For this review, take the finished solid that the model builds, in its own axes (mm). A direction names the side the tool comes from. Coordinates: 2 decimals unless noted, no trailing zeros. Loops run counter-clockwise (first coordinate to the right, second up) from the corner with the lowest first, then second, coordinate; pieces in that order, holes last.
1. Take a section at B-B, the plane x = -6.5. State the section outline as (y, z) points.
2. Clearance check with flat-ended pins moving along their axes: P1, Ø7.5, axis at y = 14, z = 48, coming from the +X side; P2, Ø1, axis at x = -1.5, z = 45, coming from the +Y side; P3, Ø10, axis at x = 8, y = -21, coming from the -Z side. State where each tip first meets the part, or that it passes through.
3. Machinability: for faces 1 (the face through (22.87, 19.61, 81.98)), 2 (the face through (15, 2.635, 16)), 3 (the face through (15, -20, 70)), 4 (the face through (14.45, -30.89, 41.74)), which of the approach directions +Z, -Z, +X, -X, +Y, -Y give a long, thin tool a straight path to every point of the face, cutting with its end or side? Answer none if there is none.
4. Mouldability with a two-part tool opening along Y and no side actions: class faces 5 (the face through (-1.51, 13.54, 49.3)), 6 (the face through (34.345, 18, 49)), 7 (the face through (29.841, 23.163, 22.211)) as pulls with the +Y half, pulls with the -Y half, needs draft (parallel to the pull), parting line crosses it, or undercut.
5. Take a section at A-A, the plane y = -27.5. State the section outline as (x, z) points.
6. Take a section at D-D, the plane z = 45.5. State the section outline as (x, y) points.
7. Take a section at C-C, the plane z = 14. State the section outline as (x, y) points.
8. To check wall thickness, follow probe 1 along Y at (x, z) = (22, 80); probe 2 along Z at (x, y) = (15, -37.5); probe 3 along Z at (x, y) = (14, -6.5). State the ranges of each line that lie inside material, in increasing order.
```python
from build123d import *

# Parameters (mm, degrees)
BOSS_EXTRUDE1_DEPTH = 100
SKETCH3_W           = 32.48675427
SKETCH3_H           = 45
CUT_EXTRUDE5_DEPTH  = 120.560658656
SKETCH7_W           = 30
SKETCH7_H           = 45
CUT_EXTRUDE7_DEPTH  = 120.560658656
SKETCH8_R           = 10
CUT_EXTRUDE8_DEPTH  = 120.560658656
SKETCH9_R           = 2.5
CUT_EXTRUDE9_DEPTH  = 13
SKETCH10_R          = 3
CUT_EXTRUDE10_DEPTH = 10
FILLET1_R           = 1
FILLET2_R           = 1
SKETCH11_R          = 2.5
CUT_EXTRUDE11_DEPTH = 13
SKETCH12_R          = 3
CUT_EXTRUDE12_DEPTH = 10
FILLET3_R           = 1


with BuildPart() as part:
    # Sketch2 → Boss-Extrude1 (new body)
    with BuildSketch(Plane.XY):
        with BuildLine():
            Line((-10.655452858, -42.364502809), (39.344547142, -42.364502809))
            Line((39.344547142, -42.364502809), (39.344547142, 2.635497191))
            Line((39.344547142, 2.635497191), (39.344547142, 5.635497191))
            Line((39.344547142, 5.635497191), (34.344547142, 5.635497191))
            Line((34.344547142, 5.635497191), (34.344547142, 30.635497191))
            Line((34.344547142, 30.635497191), (9.344547142, 30.635497191))
            ThreePointArc((9.344547142, 30.635497191), (2.27347933, 27.706565003), (-0.655452858, 20.635497191))
            Line((-0.655452858, 20.635497191), (-0.655452858, 15.635497191))
            ThreePointArc((-0.655452858, 15.635497191), (-1.534132514, 13.514176848), (-3.655452858, 12.635497191))
            Line((-3.655452858, 12.635497191), (-10.655452858, 12.635497191))
            Line((-10.655452858, 12.635497191), (-10.655452858, -42.364502809))
        make_face()
    extrude(amount=BOSS_EXTRUDE1_DEPTH)

    # Sketch3 → Cut-Extrude5 (cut, through all)
    with BuildSketch(Plane(origin=(39.344547142, 0, 0), x_dir=(0, 0, -1), z_dir=(1, 0, 0))):
        with Locations((-16.243377135, -19.864502809)):
            Rectangle(SKETCH3_W, SKETCH3_H)
    extrude(amount=-CUT_EXTRUDE5_DEPTH, mode=Mode.SUBTRACT)

    # Sketch7 → Cut-Extrude7 (cut, through all)
    with BuildSketch(Plane(origin=(39.344547142, 0, 0), x_dir=(0, 0, -1), z_dir=(1, 0, 0))):
        with Locations((-85, -19.864502809)):
            Rectangle(SKETCH7_W, SKETCH7_H)
    extrude(amount=-CUT_EXTRUDE7_DEPTH, mode=Mode.SUBTRACT)

    # Sketch8 → Cut-Extrude8 (cut, through all)
    with BuildSketch(Plane(origin=(39.344547142, 0, 0), x_dir=(0, 0, -1), z_dir=(1, 0, 0))):
        with Locations((-51.243377135, -24.364502809)):
            Circle(SKETCH8_R)
    extrude(amount=-CUT_EXTRUDE8_DEPTH, mode=Mode.SUBTRACT)

    # Sketch9 → Cut-Extrude9 (cut)
    with BuildSketch(Plane(origin=(34.344547142, 0, 0), x_dir=(0, 0, -1), z_dir=(1, 0, 0))):
        with Locations((-20, 21.135497191)):
            Circle(SKETCH9_R)
        with Locations((-80, 21.135497191)):
            Circle(SKETCH9_R)
    extrude(amount=-CUT_EXTRUDE9_DEPTH, mode=Mode.SUBTRACT)

    # Sketch10 → Cut-Extrude10 (cut)
    with BuildSketch(Plane(origin=(34.344547142, 0, 0), x_dir=(0, 0, -1), z_dir=(1, 0, 0))):
        with Locations((-20, 21.135497191)):
            Circle(SKETCH10_R)
        with Locations(Location((-80, 21.135497191, 0), (0, 0, 180))):
            Circle(SKETCH10_R)
    extrude(amount=-CUT_EXTRUDE10_DEPTH, mode=Mode.SUBTRACT)

    # Fillet1
    # the kernel refuses this fillet: 1 mm, written as the material it adds along each edge
    with BuildSketch(Plane(origin=(24.344547142, 21.135497191, 20), x_dir=(0, 0, -1), z_dir=(0, -1, 0))) as fillet1_piece_1:
        with BuildLine():
            CenterArc((2, 0.866025404), FILLET1_R, 300, 60)
            Line((2.5, 0), (2.51, -0.017320508))
            ThreePointArc((2.51, -0.017320508), (2.75, -0.02), (3, -0.02))
            Line((3, -0.02), (3.02, 0))
            Line((3.02, 0), (3.02, 0.866025404))
            Line((3.02, 0.866025404), (3, 0.866025404))
        make_face()
    revolve(axis=Axis((24.344547142, 21.135497191, 20), (1, 0, 0)))

    # Fillet2
    # the kernel refuses this fillet: 1 mm, written as the material it adds along each edge
    with BuildSketch(Plane(origin=(24.344547142, 21.135497191, 80), x_dir=(0, 0, 1), z_dir=(0, 1, 0))) as fillet2_piece_1:
        with BuildLine():
            CenterArc((2, 0.866025404), FILLET2_R, 300, 60)
            Line((2.5, 0), (2.51, -0.017320508))
            ThreePointArc((2.51, -0.017320508), (2.75, -0.02), (3, -0.02))
            Line((3, -0.02), (3.02, 0))
            Line((3.02, 0), (3.02, 0.866025404))
            Line((3.02, 0.866025404), (3, 0.866025404))
        make_face()
    revolve(axis=Axis((24.344547142, 21.135497191, 80), (1, 0, 0)))

    # Sketch11 → Cut-Extrude11 (cut)
    with BuildSketch(Plane.XZ.offset(42.364502809)):
        with Locations(Location((14.344547142, 63.243377135, 0), (0, 0, 270))):
            Circle(SKETCH11_R)
        with Locations(Location((14.344547142, 39.243377135, 0), (0, 0, 270))):
            Circle(SKETCH11_R)
    extrude(amount=-CUT_EXTRUDE11_DEPTH, mode=Mode.SUBTRACT)

    # Sketch12 → Cut-Extrude12 (cut)
    with BuildSketch(Plane.XZ.offset(42.364502809)):
        with Locations(Location((14.344547142, 63.243377135, 0), (0, 0, 270))):
            Circle(SKETCH12_R)
        with Locations(Location((14.344547142, 39.243377135, 0), (0, 0, 90))):
            Circle(SKETCH12_R)
    extrude(amount=-CUT_EXTRUDE12_DEPTH, mode=Mode.SUBTRACT)

    # Fillet3
    # the kernel refuses this fillet: 1 mm, written as the material it adds along each edge
    with BuildSketch(Plane(origin=(14.344547142, -32.364502809, 63.243377135), x_dir=(0, 0, -1), z_dir=(-1, 0, 0))) as fillet3_piece_1:
        with BuildLine():
            CenterArc((2, 0.866025404), FILLET3_R, 300, 60)
            Line((2.5, 0), (2.51, -0.017320508))
            ThreePointArc((2.51, -0.017320508), (2.75, -0.02), (3, -0.02))
            Line((3, -0.02), (3.02, 0))
            Line((3.02, 0), (3.02, 0.866025404))
            Line((3.02, 0.866025404), (3, 0.866025404))
        make_face()
    revolve(axis=Axis((14.344547142, -32.364502809, 63.243377135), (0, -1, 0)))
    with BuildSketch(Plane(origin=(14.344547142, -32.364502809, 39.243377135), x_dir=(0, 0, 1), z_dir=(1, 0, 0))) as fillet3_piece_2:
        with BuildLine():
            CenterArc((2, 0.866025404), FILLET3_R, 300, 60)
            Line((2.5, 0), (2.51, -0.017320508))
            ThreePointArc((2.51, -0.017320508), (2.75, -0.02), (3, -0.02))
            Line((3, -0.02), (3.02, 0))
            Line((3.02, 0), (3.02, 0.866025404))
            Line((3.02, 0.866025404), (3, 0.866025404))
        make_face()
    revolve(axis=Axis((14.344547142, -32.364502809, 39.243377135), (0, -1, 0)))


solid = part.part
```
Results list:
1. outline: (-42.36, 32.49) - (2.64, 32.49) - (2.64, 0) - (12.64, 0) - (12.64, 100) - (2.64, 100) - (2.64, 70) - (-42.36, 70) - close; hole circle Ø20 at (-24.36, 51.24)
2. P1: stops at x = 34.34
2. P2: stops at y = 14.24
2. P3: stops at z = 32.49
3. face 1: +X
3. face 2: -Z, +X, -X, -Y
3. face 3: +Z, +X, -X, -Y
3. face 4: -Y
4. face 5: pulls with the +Y half
4. face 6: needs draft
4. face 7: undercut
5. outline: (-10.66, 32.49) - (39.34, 32.49) - (39.34, 41.75) - (-10.66, 41.75) - close; (-10.66, 60.74) - (39.34, 60.74) - (39.34, 70) - (-10.66, 70) - close
6. outline: (-10.66, -42.36) - (39.34, -42.36) - (39.34, -32.55) - (-10.66, -32.55) - close; (-10.66, -16.18) - (39.34, -16.18) - (39.34, 5.64) - (34.34, 5.64) - (34.34, 30.64) - (9.34, 30.64) arc R10 ccw to (-0.66, 20.64) - (-0.66, 15.64) arc R3 cw to (-3.66, 12.64) - (-10.66, 12.64) - close
7. outline: (-10.66, 2.64) - (39.34, 2.64) - (39.34, 5.64) - (34.34, 5.64) - (34.34, 30.64) - (9.34, 30.64) arc R10 ccw to (-0.66, 20.64) - (-0.66, 15.64) arc R3 cw to (-3.66, 12.64) - (-10.66, 12.64) - close
8. probe 1: y = 2.64 to 18.64, 23.64 to 30.64
8. probe 2: z = 32.49 to 36.32, 42.17 to 60.32, 66.17 to 70
8. probe 3: z = 32.49 to 70
